```python
from build123d import *

# Parameters (mm, degrees)
CUT_EXTRUDE_1_DEPTH       = 2
CUT_EXTRUDE_START         = 9
CUT_EXTRUDE_1_2_OUTLINE_W = 2
CUT_EXTRUDE_1_2_OUTLINE_H = 19
CUT_EXTRUDE_1_2_DEPTH     = 4
CUT_EXTRUDE_START_2       = 2
CUT_EXTRUDE_1_3_OUTLINE_W = 2
CUT_EXTRUDE_1_3_OUTLINE_H = 19
CUT_EXTRUDE_1_3_DEPTH     = 2
CUT_EXTRUDE_START_3       = -49.585786703
CUT_EXTRUDE_1_4_DEPTH     = 2
CUT_EXTRUDE_START_4       = -5.128602194
CUT_EXTRUDE_1_5_DEPTH     = 19
SKETCH_3_W                = 100.571067812
SKETCH_3_H                = 17.071067812
EXTRUDE_1_DEPTH           = 1
CUT_EXTRUDE_2_REACH       = 75.102
SKETCH_4_W                = 17
SKETCH_4_H                = 14
SKETCH_5_W                = 8
SKETCH_5_H                = 5
SKETCH_5_W_2              = 47
SKETCH_5_H_2              = 1.571067812
EXTRUDE_2_DEPTH           = 8.2
CUT_EXTRUDE_3_REACH       = 75.563
SKETCH_6_R                = 1.5
FILLET_1_R                = 1
FILLET_2_R                = 3
SKETCH_8_W                = 7
SKETCH_8_H                = 10
CUT_EXTRUDE_4_DEPTH       = 1
FILLET_3_R                = 1


with BuildPart() as part:
    # 切除-拉伸1: read off the stored shape, not the designer's step
    # 切除-拉伸1 outline → 切除-拉伸1 (new body)
    with BuildSketch(Plane.XY):
        Polygon((-49.585786703, 13.871397806), (-49.585786703, -5.128602194), (-46.085786703, -5.128602194), (-41.32842739, -0.371242882), (59.242640422, -0.371242882), (62.778174328, 3.164291024), (69.778174328, 3.164291024), (69.778174328, 13.164291024), (62.778174328, 13.164291024), (59.242640422, 16.69982493), (-43.257359578, 16.69982493), (-46.085786703, 13.871397806), align=None)
    extrude(amount=CUT_EXTRUDE_1_DEPTH)

    # Cut-Extrude 1 3 outline → Cut-Extrude 1 3 (add)
    with BuildSketch(Plane.XY.offset(CUT_EXTRUDE_START_2)):
        with Locations((-48.585786703, 4.371397806)):
            Rectangle(CUT_EXTRUDE_1_3_OUTLINE_W, CUT_EXTRUDE_1_3_OUTLINE_H)
    extrude(amount=CUT_EXTRUDE_1_3_DEPTH)



with BuildPart() as body_2:
    # Cut-Extrude 1 2 outline → Cut-Extrude 1 2 (new body)
    with BuildSketch(Plane.XY.offset(CUT_EXTRUDE_START)):
        with Locations((-48.585786703, 4.371397806)):
            Rectangle(CUT_EXTRUDE_1_2_OUTLINE_W, CUT_EXTRUDE_1_2_OUTLINE_H)
    extrude(amount=CUT_EXTRUDE_1_2_DEPTH)


with BuildPart() as part_1:
    add(part.part)

    add(body_2.part)  # Cut-Extrude 1 4 merges body 2
    # Cut-Extrude 1 4 outline → Cut-Extrude 1 4 (add)
    with BuildSketch(Plane.YZ.offset(CUT_EXTRUDE_START_3)):
        with BuildLine():
            Line((13.871397806, 9), (-2.628602194, 9))
            ThreePointArc((-2.628602194, 9), (-0.128602194, 6.5), (-2.628602194, 4))
            Line((-2.628602194, 4), (13.871397806, 4))
            Line((13.871397806, 4), (13.871397806, 9))
        make_face()
    extrude(amount=CUT_EXTRUDE_1_4_DEPTH)

    # Cut-Extrude 1 5 outline → Cut-Extrude 1 5 (add)
    with BuildSketch(Plane(origin=(0, 0, 0), x_dir=(1, 0, 0), z_dir=(0, 1, 0)).offset(CUT_EXTRUDE_START_4)):
        with BuildLine():
            ThreePointArc((-47.585786703, -3), (-47.292893484, -2.292893219), (-46.585786703, -2))
            Line((-46.585786703, -2), (-47.585786703, -2))
            Line((-47.585786703, -2), (-47.585786703, -3))
        make_face()
    extrude(amount=CUT_EXTRUDE_1_5_DEPTH)

    # 草图3 → 凸台-拉伸1 (add)
    with BuildSketch(Plane(origin=(0, 0, 0), x_dir=(-1, 0, 0), z_dir=(0, 0, -1))):
        with Locations((-8.957106516, 8.164291024)):
            Rectangle(SKETCH_3_W, SKETCH_3_H)
    extrude(amount=EXTRUDE_1_DEPTH)

    # 草图4 → 切除-拉伸2 (cut, up to next)
    with BuildSketch(Plane(origin=(0, 0, -1), x_dir=(-1, 0, 0), z_dir=(0, 0, -1)), mode=Mode.PRIVATE) as cut_extrude_2_sk1:
        with Locations((-8.67157261, 8.19982493)):
            Rectangle(SKETCH_4_W, SKETCH_4_H)
    cut_extrude_2_tool1 = extrude(cut_extrude_2_sk1.sketch, amount=-CUT_EXTRUDE_2_REACH, mode=Mode.PRIVATE) & part_1.part
    add(cut_extrude_2_tool1.solids().sort_by_distance((8.671573, 8.199825, -1))[0], mode=Mode.SUBTRACT)

    # 草图5 → 凸台-拉伸2 (add)
    with BuildSketch(Plane(origin=(0, 0, -1), x_dir=(-1, 0, 0), z_dir=(0, 0, -1))):
        with Locations((-24.67157261, 11.69982493)):
            Rectangle(SKETCH_5_W, SKETCH_5_H)
        with Locations((7.32842739, 11.69982493)):
            Rectangle(SKETCH_5_W, SKETCH_5_H)
        with Locations((-8.67157261, 0.414291024)):
            Rectangle(SKETCH_5_W_2, SKETCH_5_H_2)
    extrude(amount=EXTRUDE_2_DEPTH)

    # 草图6 → 切除-拉伸3 (cut, up to next)
    with BuildSketch(Plane(origin=(0, 14.19982493, 0), x_dir=(1, 0, 0), z_dir=(0, 1, 0)), mode=Mode.PRIVATE) as cut_extrude_3_sk1:
        with Locations(Location((-7.32842739, 5.2, 0), (0, 0, 270))):
            Circle(SKETCH_6_R)
    cut_extrude_3_tool1 = extrude(cut_extrude_3_sk1.sketch, amount=-CUT_EXTRUDE_3_REACH, mode=Mode.PRIVATE) & part_1.part
    # 草图6 → 切除-拉伸3 (cut, up to next)
    with BuildSketch(Plane(origin=(0, 14.19982493, 0), x_dir=(1, 0, 0), z_dir=(0, 1, 0)), mode=Mode.PRIVATE) as cut_extrude_3_sk2:
        with Locations(Location((24.67157261, 5.2, 0), (0, 0, 270))):
            Circle(SKETCH_6_R)
    cut_extrude_3_tool2 = extrude(cut_extrude_3_sk2.sketch, amount=-CUT_EXTRUDE_3_REACH, mode=Mode.PRIVATE) & part_1.part
    add(cut_extrude_3_tool1.solids().sort_by_distance((-7.328427, 14.199825, -5.2))[0], mode=Mode.SUBTRACT)
    add(cut_extrude_3_tool2.solids().sort_by_distance((24.671573, 14.199825, -5.2))[0], mode=Mode.SUBTRACT)

    # 圆角1
    fillet_1_edges = [part_1.edges().sort_by_distance(p)[0] for p in [
        (59.242640422, 8.164291024, 0),
        (-41.32842739, 8.164291024, 0),
    ]]
    fillet(fillet_1_edges, radius=FILLET_1_R - 0.0001)  # a hair under: the kernel refuses the full size

    # 圆角2
    fillet_2_edges = [part_1.edges().sort_by_distance(p)[0] for p in [
        (-7.32842739, 1.19982493, -1),
        (24.67157261, 1.19982493, -1),
    ]]
    fillet(fillet_2_edges, radius=FILLET_2_R)

    # 草图8 → 切除-拉伸4 (cut)
    with BuildSketch(Plane(origin=(0, 0, 0), x_dir=(-1, 0, 0), z_dir=(0, 0, -1))):
        with Locations((-66.278174328, 8.164291024)):
            Rectangle(SKETCH_8_W, SKETCH_8_H)
    extrude(amount=-CUT_EXTRUDE_4_DEPTH, mode=Mode.SUBTRACT)

    # 圆角3
    fillet_3_edges = [part_1.edges().sort_by_distance(p)[0] for p in [
        (62.778174328, 8.164291024, 1),
    ]]
    fillet(fillet_3_edges, radius=FILLET_3_R - 0.0001)  # a hair under: the kernel refuses the full size


solid = part_1.part
```
Model file for the job. Use its own axes, mm. A direction names the side the tool comes from. Coordinates: 2 decimals unless noted, no trailing zeros. Order: outer loops, then holes, each group sorted by start corner. A loop starts at its lowest first (then second) coordinate and runs counter-clockwise, first axis right, second up. Notation, with made-up numbers: (-36, -2.5) -> (12, -2.5) arc R28 ccw to (12, 36.5) -> close; hole circle Ø4 at (84, -0.75). An arc over 180 degrees is marked (long way). Answer as a JSON object with one key per item and string values. Group by question number.
1) Cut at C-C, the plane x = 30. Write the cut outline in (y, z), then the cut area to 3 significant figures.
2) Pull direction Y, two halves, no side cores. Call faces 4 (the face through (-44.65, 15.31, 0.99)), 5 (the face through (0.172, 8, 0)), 6 (the face through (-11.328, 12, -5)): +Y half, -Y half, draft (parallel to the pull), parting line (faces both ways), or undercut.
3) Drill centre lines: L1, parallel to X at y = 11.6, z = -5.2; L2, parallel to X at y = 10.25, z = -4; L3, parallel to Z at x = 21, y = 12.5. Where is each one in solid material? Low to high.
4) Flat gauge pins, fed straight in: pin 1 (1 mm diameter, centred on x = -7.5, z = -5, fed in from +Y); pin 2 (9 mm diameter, centred on x = 18, z = -4.5, fed in from -Y); pin 3 (5 mm diameter, centred on x = 66.5, y = 10, fed in from -Z); pin 4 (10 mm diameter, centred on x = 11, z = 10.5, fed in from +Y). Where does each tip first touch, or does it go through?
5) Cut at B-B, the plane z = -5.2. Write the cut outline in (x, y).
6) Which spindle directions (+Z, -Z, +X, -X, +Y, -Y) get a long thin tool onto all of the face, cutting with end or side? Do faces 1 (the face through (27, 14.2, -5)), 2 (the face through (17.172, 8, 0)), 3 (the face through (-49, 13.871, 6)). Say none if no direction does.
7) Cut at D-D, the plane z = 11.25. Write the cut outline in (x, y), then the cut area to 3 significant figures.
Check values:
{
 "1": {"outline": "(-0.37, -9.2) -> (1.2, -9.2) -> (1.2, -4) arc R3 cw to (4.2, -1) -> (16.7, -1) -> (16.7, 2) -> (-0.37, 2) -> close", "area": "66.0 mm²"},
 "2": {"face 4": "+Y half", "face 5": "undercut", "face 6": "draft"},
 "3": {"L1": "x = -11.33 to -8.83, -5.83 to -3.33, 20.67 to 23.17, 26.17 to 28.67", "L2": "x = -11.33 to -8.23, -6.43 to -3.33, 20.67 to 23.77, 25.57 to 28.67", "L3": "z = -9.2 to 2"},
 "4": {"pin 1": "stops at y = 1.2", "pin 2": "stops at y = -0.37", "pin 3": "stops at z = 1", "pin 4": "passes through"},
 "5": {"outline": "(-14.83, -0.37) -> (32.17, -0.37) -> (32.17, 1.2) -> (-14.83, 1.2) -> close; (-11.33, 9.2) -> (-8.83, 9.2) -> (-8.83, 14.2) -> (-11.33, 14.2) -> close; (-5.83, 9.2) -> (-3.33, 9.2) -> (-3.33, 14.2) -> (-5.83, 14.2) -> close; (20.67, 9.2) -> (23.17, 9.2) -> (23.17, 14.2) -> (20.67, 14.2) -> close; (26.17, 9.2) -> (28.67, 9.2) -> (28.67, 14.2) -> (26.17, 14.2) -> close"},
 "6": {"face 1": "-Z, +X, -X, +Y", "face 2": "+Z, -Z", "face 3": "+Z, -Z, -X, +Y"},
 "7": {"outline": "(-49.59, -5.13) -> (-47.59, -5.13) -> (-47.59, 13.87) -> (-49.59, 13.87) -> close", "area": "38.0 mm²"}
}
